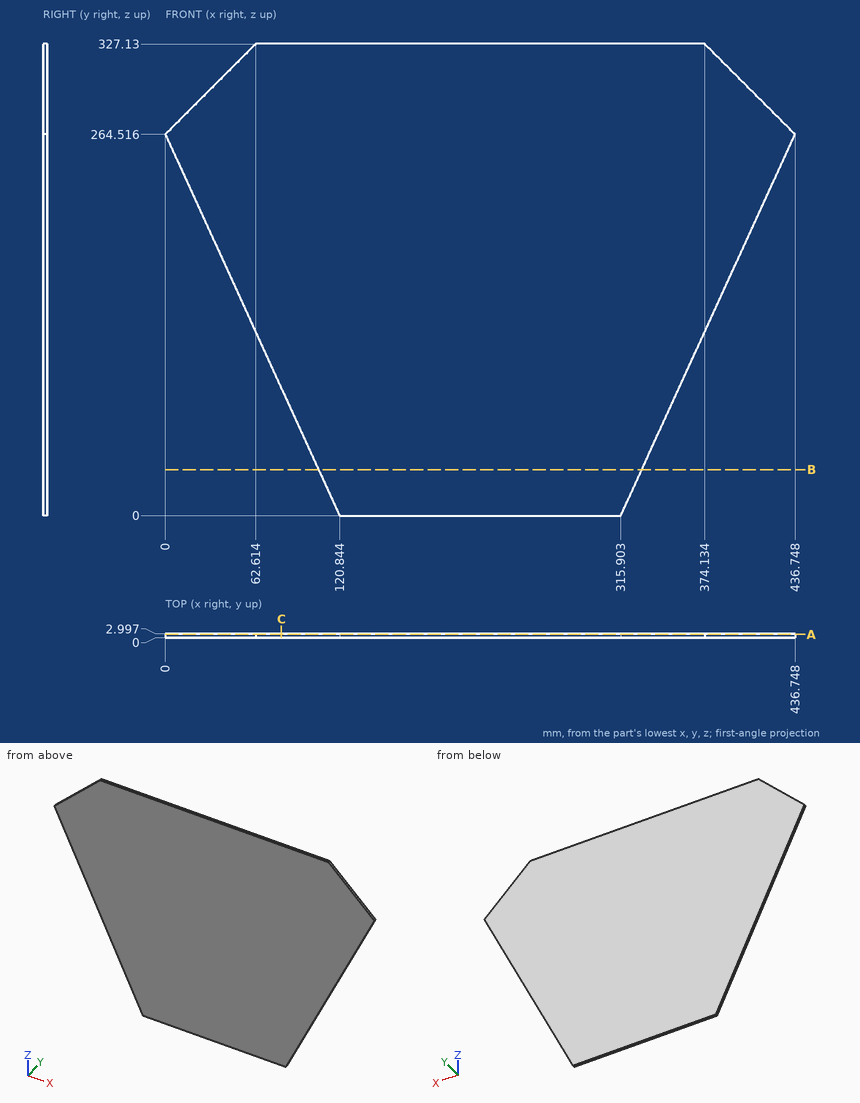
For this review, use the dimensioned drawing (mm, ordinates from the lowest corner) and the shaded views. Coordinates: 2 decimals unless noted, no trailing zeros. Write each loop counter-clockwise with the first axis right and the second up, starting at its lowest first coordinate (ties: lowest second). Pieces come first, ordered by that corner, then holes. Notation, with made-up numbers: (88, 13.5) -> (131, 13.5) arc R17 ccw to (131, 33.5) -> close; hole circle Ø6 at (83, 28.25). An arc over 180 degrees is marked (long way). Write each question's results on one line, items separated by ' | '. Start each with the question number.
(1) For line 1 along Z through (x, y) = (43, 2.3) (1 decimal); line 2 along Z through (x, y) = (341.5, 0.8) (1 decimal); line 3 along X through (y, z) = (0.9, 302.5) (1 decimal), list the stretches that pass through material, from the lowest coordinate up. Write a range as from..to.
(2) Take a section at C-C on x = 80.5. Write out the cut boundary in (y, z).
(3) Take a section at B-B on z = 32. Write out the cut boundary in (x, y) (1 decimal).
(4) Take a section at A-A on y = 2.45. Write out the cut boundary in (x, z) (1 decimal), and give its area (3 significant figures).
Results found:
1) line 1: z = 170.4..307.5 | line 2: z = 56..327.1 | line 3: x = 38..398.8
2) outline: (0, 88.31) -> (3, 88.31) -> (3, 327.13) -> (0, 327.13) -> close
3) outline: (106.2, 0) -> (330.5, 0) -> (330.5, 3) -> (106.2, 3) -> close
4) outline: (0, 264.5) -> (120.8, 0) -> (315.9, 0) -> (436.7, 264.5) -> (374.1, 327.1) -> (62.6, 327.1) -> close | area: 107,000 mm2
